Autodesk Inventor part; units mm, degrees
ref_plane "Płaszczyzna konstrukcyjna2" through (0, -18.3848, 0) normal (0, -1, 0) x (1, 0, 0)
ref_plane "YZ Plane" through (0, 0, 0) normal (1, 0, 0) x (0, 1, 0)
ref_plane "XZ Plane" through (0, 0, 0) normal (0, 1, 0) x (-1, 0, 0)
sketch "Szkic6" plane through (0, 0, 0) normal (0, 0, 1) x (1, 0, 0)
  line L0 (-29.6067, 0) -> (35.2678, 0) construction
  line L1 (0, 42.3419) -> (0, -58.3726) construction
  arc A0 (7.6152, 0) -> (0, -18.3848) centre (26, -18.3848) ccw
  line L2 (0, -18.3848) -> (26, -18.3848) construction
  line L3 (26, -18.3848) -> (-20.3389, 27.9541) construction
  line L4 (7.6152, 0) -> (25.7172, 18.1019)
  line L5 (0, -18.3848) -> (0, -43.9848)
  point P0 (0, 0)
  dimension "d24" = 55
  dimension "d31" = 45
  dimension "d36" = 0
  dimension "d37" = 0
ref_plane "Płaszczyzna konstrukcyjna2" through (0, -18.3848, 0) normal (0, -1, 0) x (1, 0, 0)
sketch "Szkic8" plane through (0, -18.3848, 0) normal (0, -1, 0) x (1, 0, 0)
  circle A0 centre (0, 0) radius 6.5
  circle A1 centre (0, 0) radius 5
  dimension "d32" = 34
  dimension "d33" = 1.5
sweep "Przeciągnięcie2" add profiles "Szkic8" path "Szkic6"
equation "\"d32\" = OD"
equation "\"d33\" = THK"
equation "\"d24\" = R"
equation "\"d31\" = KAT"
equation "\"SzerokośćGięciaPodcięcia\" = Grubość"
equation "\"RozmiarPodcięciaNarożnika\" = 4 * Grubość"
equation "\"PromieńPrzejścia\" = PromieńGięcia"
equation "\"Rozmiar_promienia_Jacobiego\" = PromieńGięcia"
equation "\"Wielk_odstępu\" = Grubość"
equation "\"d2\" = PromieńGięcia"
equation "\"d23\" = PromieńGięcia"
equation "\"R\" = 55"
equation "\"OD\" = 34"
equation "\"THK\" = 1.5"
equation "\"KAT\" = 45deg"
equation "\"PROSTKA\" = 0"
properties part number "Kolano 45° ø34x1,5 R55" material "304L"
Could you check a few things on this model? Use its own coordinates, in mm. Round coordinates to 2 decimals unless told otherwise and drop trailing zeros. Loops run counter-clockwise (first coordinate to the right, second up) from the corner with the lowest first, then second, coordinate; pieces in that order, holes last. Notation, with made-up numbers: (66.25, 72) - (94.25, 72) arc R14 ccw to (94.25, 95) - close; hole circle Ø7 at (41, 22). An arc over 180 degrees is marked (long way). Answer in a Markdown table with one row per item. Add a question column.
(1) If we section it at A-A (y = -28): Please give me the cut outline in (x, z).
(2) I'm going to push flat-ended pins straight in: pin 1 (4 mm diameter, centred on y = 6.5, z = -4, fed in from +X); pin 2 (2 mm diameter, centred on y = 10, z = 0, fed in from +X); pin 3 (4 mm diameter, centred on y = -10, z = 2.5, fed in from +X). Where does each tip first touch, or does it pass through?
(3) I need wall thicknesses on line 1 along Z through (x, y) = (0, -28); line 2 along X through (y, z) = (-32.5, -1); line 3 along Y through (x, z) = (17.5, -3.75). Which ranges of each line are inside material? Lowest first, please.
(4) If we mould it in two halves opening along Z, with no side actions, what happens to faces 1 (the face through (-1.08, -31.36, -4.88)), 2 (the face through (-5, -43.985, -2)), 3 (the face through (-5.158, -31.364, -3.955))? For each: pulls with the +Z half, pulls with the -Z half, needs draft (parallel to the pull), parting line crosses it, or undercut.
Model answer:
| question | item | result |
|---|---|---|
| 1 | outline | circle Ø13 at (0, 0); hole circle Ø10 at (0, 0) |
| 2 | pin 1 | stops at x = 24.01 |
| 2 | pin 2 | stops at x = 27.81 |
| 2 | pin 3 | stops at x = 9.13 |
| 3 | line 1 | z = -6.5 to -5, 5 to 6.5 |
| 3 | line 2 | x = -6.42 to -4.9, 4.9 to 6.42 |
| 3 | line 3 | y = 2.38 to 5.21, 14.56 to 17.39 |
| 4 | face 1 | undercut |
| 4 | face 2 | needs draft |
| 4 | face 3 | parting line crosses it |
